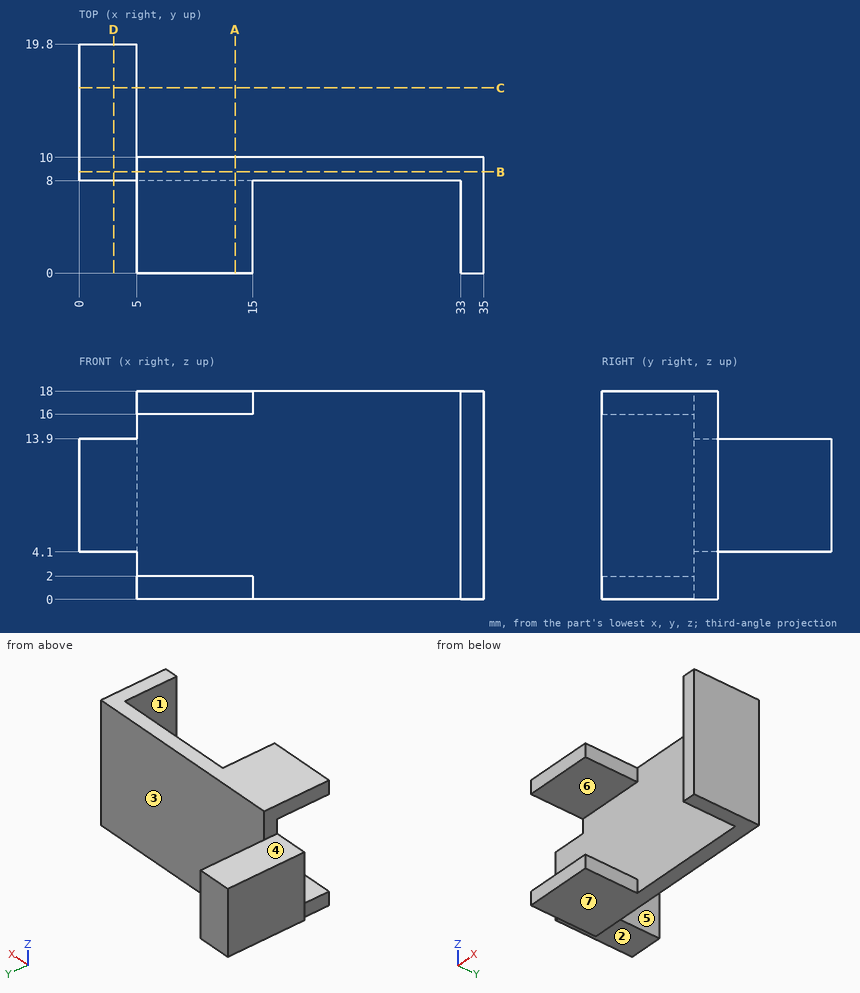
The drawing under review shows one solid part. Ordinate dimensions are in mm from its lowest x, y, z. A direction names the side the tool comes from. Coordinates: 2 decimals unless noted, no trailing zeros. Write each loop counter-clockwise with the first axis right and the second up, starting at its lowest first coordinate (ties: lowest second). Pieces come first, ordered by that corner, then holes. Notation, with made-up numbers: (86, 44.25) -> (130, 44.25) arc R14 ccw to (130, 55.25) -> close; hole circle Ø4 at (-19, 56). An arc over 180 degrees is marked (long way). One line per item, written item: value. Start each with the question number.
Q1. The part is to be moulded in two halves that separate along Z. For the marked faces 4, 5, 6 and 7, say which applies: +Z half, -Z half, draft (parallel to the pull), parting line (faces both ways), or undercut.
Q2. Add section D-D, the plane x = 3. Give the boundary of the cut face in (y, z).
Q3. Add section C-C, the plane y = 16. Give the boundary of the cut face in (x, z).
Q4. Add section A-A, the plane x = 13.5. Give the boundary of the cut face in (y, z), then the cut area to 3 significant figures.
Q5. For the marked faces 1, 2 and 3, list the 3-axis set-ups (+Z, -Z, +X, -X, +Y, -Y) from which the entire face can be reached by the end or side of a thin tool; tool diameter is ignored.
Q6. Add section B-B, the plane y = 8.75. Give the boundary of the cut face in (x, z), then the cut area to 3 significant figures.
Q7. To check wall thickness, follow probe 1 along Z at (x, y) = (6, 2.5); probe 2 along Y at (x, z) = (30, 11.25); probe 3 along Y at (x, z) = (10, 16.25). State the ranges of each line that lie inside material, in increasing order.
Q8. Clearance check with flat-ended pins moving along their axes: P1, Ø10, axis at x = 24, z = 4, coming from the +Y side; P2, Ø4, axis at y = 2, z = 5, coming from the -X side; P3, Ø1, axis at x = 18.5, z = 12, coming from the -Y side. State where each tip first meets the part, or that it passes through.
Response:
1. face 4: +Z half
1. face 5: draft
1. face 6: undercut
1. face 7: -Z half
2. outline: (8, 4.1) -> (19.8, 4.1) -> (19.8, 13.9) -> (8, 13.9) -> close
3. outline: (0, 4.1) -> (5, 4.1) -> (5, 13.9) -> (0, 13.9) -> close
4. outline: (0, 0) -> (10, 0) -> (10, 18) -> (0, 18) -> (0, 16) -> (8, 16) -> (8, 2) -> (0, 2) -> close
4. area: 68.0 mm²
5. face 1: +Z, -Z, -Y
5. face 2: -Z, -X, +Y, -Y
5. face 3: +Z, -Z, +X, +Y
6. outline: (0, 4.1) -> (5, 4.1) -> (5, 0) -> (35, 0) -> (35, 18) -> (5, 18) -> (5, 13.9) -> (0, 13.9) -> close
6. area: 589 mm²
7. probe 1: 0 to 2, 16 to 18
7. probe 2: 8 to 10
7. probe 3: 0 to 10
8. P1: y = 10
8. P2: x = 33
8. P3: y = 8
